Design review of the part built by this model. Coordinates are the model's own, in mm. Coordinates: 2 decimals unless noted, no trailing zeros. Loops run counter-clockwise (first coordinate to the right, second up) from the corner with the lowest first, then second, coordinate; pieces in that order, holes last. Notation, with made-up numbers: (27.5, 86) - (75.5, 86) arc R37 cw to (75.5, 122) - close; hole circle Ø7 at (-2.5, 48). An arc over 180 degrees is marked (long way). Return JSON: item names as keys, results as strings. Group by question number.
Autodesk Inventor part; units mm, degrees
ref_plane "YZ Plane" through (0, 0, 0) normal (1, 0, 0) x (0, 1, 0)
ref_plane "XY Plane" through (0, 0, 0) normal (0, 0, 1) x (1, 0, 0)
ref_plane "Work Plane1" through (0, 35, 0) normal (0, 1, 0) x (-1, 0, 0)
ref_plane "Work Plane2" through (0, -35, 0) normal (0, 1, 0) x (-1, 0, 0)
sketch "Sketch3" plane through (0, 0, 0) normal (0, 1, 0) x (-1, 0, 0)
  line L0 (161.3, -117.07) -> (-52.7, -117.07)
  line L1 (-52.7, -117.07) -> (-52.7, 64.93)
  line L2 (-52.7, 64.93) -> (161.3, 64.93)
  line L3 (161.3, 64.93) -> (161.3, -117.07)
  circle A0 centre (0, 0) radius 37.5
  dimension "d8" = 182
  dimension "d9" = 214
  dimension "d10" = 52.7
  dimension "d11" = 64.93
  dimension "d14" = 75
extrude "Extrusion1" add sketch "Sketch3" along normal mid plane 4
sketch "Sketch4" plane through (0, 35, 0) normal (0, 1, 0) x (-1, 0, 0)
  circle A0 centre (0, 0) radius 37.5
  circle A1 centre (0, 0) radius 42.5
  dimension "d15" = 75
  dimension "d16" = 85
extrude "Extrusion2" add sketch "Sketch4" against normal up to surface (70 mm away)
sketch "Sketch5" plane through (0, -35, 0) normal (0, 1, 0) x (-1, 0, 0)
  circle A0 centre (0, 0) radius 37.5
  circle A1 centre (0, 0) radius 20
  dimension "d19" = 75
  dimension "d20" = 40
extrude "Extrusion3" add sketch "Sketch5" along normal blind 3
sketch "Sketch6" plane through (0, 0, 0) normal (0, 0, 1) x (1, 0, 0)
  line L0 (-37.5, -32) -> (37.5, -32)
  line L1 (-42.5, -35) -> (42.5, -35)
  arc A0 (-24.5305, -32) -> (-20, -35) centre (-2.9998, -4.406) ccw
  line L2 (-24.5305, -32) -> (-20, -32)
  line L3 (-20, -35) -> (-20, -32)
  line L4 (-20, -32) -> (-20, -35)
  line L5 (-24.5305, -32) -> (-20, -32)
  line L6 (0, -42.1057) -> (0, 7.0176)
  point P0 (0, 0)
  dimension "d23" = 35
  dimension "d24" = 4.5305
revolve "Revolution1" cut sketch "Sketch6" angle 360 about axis through (0, -10, 0) along (0, 1, 0) contours L0 L3 A0
sketch "Sketch7" plane through (0, 2, 0) normal (0, 1, 0) x (1, 0, 0)
  circle A0 centre (0, 0) radius 42.5
  circle A1 centre (0, 0) radius 42.5
  dimension "d26" = 85
extrude "Extrusion4" cut sketch "Sketch7" along normal mid plane 80
properties part number "tapa_lanzador_pelota"
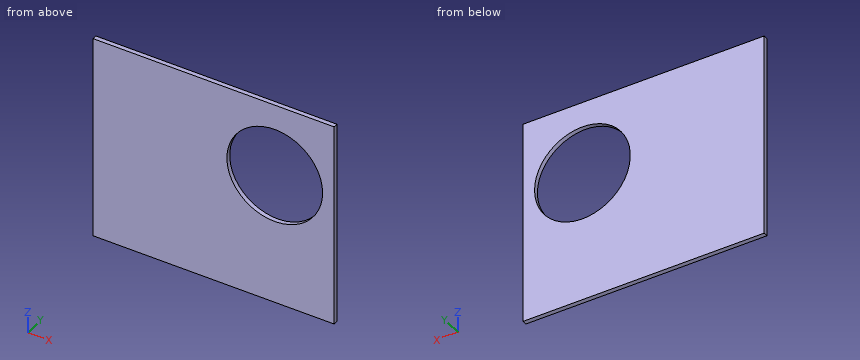
Item 1: To check wall thickness, follow line 1 (Z direction, x = 0, y = 0.7); line 2 (X direction, y = -1, z = 0); line 3 (X direction, y = 0.7, z = 36). State the ranges of each line that lie inside material, in increasing order. Write a range as from..to.
Item 2: Add section C-C (y = -0.05). State the section outline as (x, z) points, then the cut area to 3 significant figures.
Item 3: Add section A-A (x = -20). State the section outline as (y, z) points.
Item 4: Add section B-B (z = 0). State the section outline as (x, y) points.
Answers below:
{
 "1": {"line 1": "z = -117.07..-42.5, 42.5..64.93", "line 2": "x = -161.3..-42.5, 42.5..52.7", "line 3": "x = -161.3..-22.59, 22.59..52.7"},
 "2": {"outline": "(-161.3, -117.07) - (52.7, -117.07) - (52.7, 64.93) - (-161.3, 64.93) - close; hole circle Ø85 at (0, 0)", "area": "33,300 mm^2"},
 "3": {"outline": "(-2, -117.07) - (2, -117.07) - (2, -37.5) - (-2, -37.5) - close; (-2, 37.5) - (2, 37.5) - (2, 64.93) - (-2, 64.93) - close"},
 "4": {"outline": "(-161.3, -2) - (-42.5, -2) - (-42.5, 2) - (-161.3, 2) - close; (42.5, -2) - (52.7, -2) - (52.7, 2) - (42.5, 2) - close"}
}
